Work out the finished part from the listing and answer in its coordinate system (mm). Face numbers are marked on the shaded views. Give positions to 0.01 mm unless a question says otherwise; leave off trailing zeros. Write each loop counter-clockwise with the first axis right and the second up, starting at its lowest first coordinate (ties: lowest second). Pieces come first, ordered by that corner, then holes. Notation, with made-up numbers: (-21, -27.5) - (13, -27.5) arc R20 ccw to (13, -5.5) - close; hole circle Ø4 at (24, 9.25). An arc over 180 degrees is marked (long way). Write each question's results on one line, items separated by ' | '. Start each with the question number.
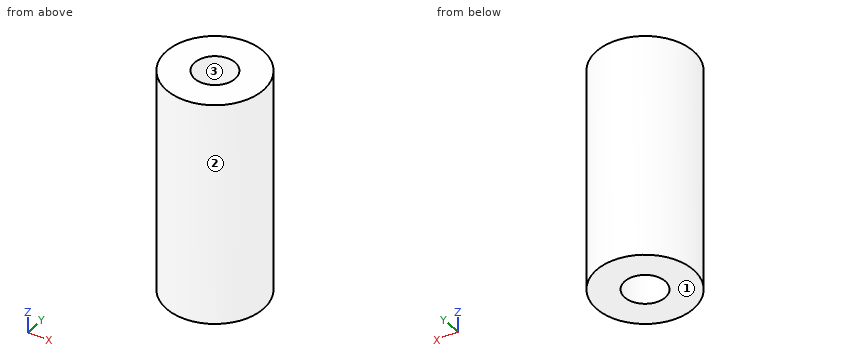
from build123d import *

# Parameters (mm, degrees)
F0_R     = 27.480462
F0_R_2   = 11.475205
F1_DEPTH = 127
F2_R     = 26.7589
F3_DEPTH = 38.1


with BuildPart() as f1:
    # F0 (on Top) → F1 (new body)
    with BuildSketch(Plane.XY):
        Circle(F0_R)
        Circle(F0_R_2, mode=Mode.SUBTRACT)
    extrude(amount=F1_DEPTH)


with BuildPart() as f3:
    # F2 (on Front) → F3 (new body, symmetric)
    with BuildSketch(Plane.XZ):
        with Locations((-124.147885, 27.501423)):
            Circle(F2_R)
    extrude(amount=F3_DEPTH, both=True)


solid = f1.part
Q1. A cutting plane is placed at D-D, the plane y = -18.5. Write down the section's boundary in (x, z).
Q2. Given pin 1 (6 mm diameter, centred on x = -19.5, z = 17, fed in from -Y); pin 2 (4 mm diameter, centred on x = -5.5, z = 75.5, fed in from -Y); pin 3 (4 mm diameter, centred on x = 17.5, z = 73, fed in from -Y), each flat-ended and moving along its own axis, determine where each tip first touches the part or whether it passes through.
Q3. The mould has two halves that part along X. Classify the marked faces 1, 2 and 3: pulls with the +X half, pulls with the -X half, needs draft (parallel to the pull), parting line crosses it, or undercut.
Q4. Consider L1, parallel to Y at x = 0, z = 95; L2, parallel to X at y = -4, z = 14; L3, parallel to Y at x = 9, z = 39. Determine where each line is inside the solid, lowest interval first.
Q5. A cutting plane is placed at C-C, the plane z = 26.5. Write down the section's boundary in (x, y).
Q6. A cutting plane is placed at A-A, the plane x = 0. Write down the section's boundary in (y, z).
Result:
1) outline: (-20.32, 0) - (20.32, 0) - (20.32, 127) - (-20.32, 127) - close
2) pin 1: stops at y = -21.98 | pin 2: stops at y = -27.26 | pin 3: stops at y = -22.69
3) face 1: needs draft | face 2: parting line crosses it | face 3: undercut
4) L1: y = -27.48 to -11.48, 11.48 to 27.48 | L2: x = -27.19 to -10.76, 10.76 to 27.19 | L3: y = -25.96 to -7.12, 7.12 to 25.96
5) outline: circle Ø54.96 at (0, 0); hole circle Ø22.95 at (0, 0)
6) outline: (-27.48, 0) - (-11.48, 0) - (-11.48, 127) - (-27.48, 127) - close; (11.48, 0) - (27.48, 0) - (27.48, 127) - (11.48, 127) - close
